Input: dimensioned drawing with shaded views. Units: mm. Origin: part minimum x, y, z. Coordinates: 2 decimals unless noted, no trailing zeros. Loops run counter-clockwise (first coordinate to the right, second up) from the corner with the lowest first, then second, coordinate; pieces in that order, holes last.
Item 1: Section A-A on z = 21. Return loops of the section in (x, y) (1 decimal).
Item 2: Ray query, line 1 along X through (y, z) = (1.5, 52); line 2 along Z through (x, y) = (35.5, 6.5) (1 decimal); line 3 along Z through (x, y) = (39, 3). Return the intervals inside material, ascending.
Item 3: Section B-B on y = 1.5. Give the number of separate pieces and of enclosed holes in the cut face.
Item 4: Section C-C on z = 96. Return loops of the section in (x, y) (1 decimal), and give its area (3 significant figures).
Item 5: Pull-direction query (Z, two-part tool) for the marked faces 1, 2 and 3; classes: released by +Z, released by -Z, zero draft, split by the parting line, or undercut.
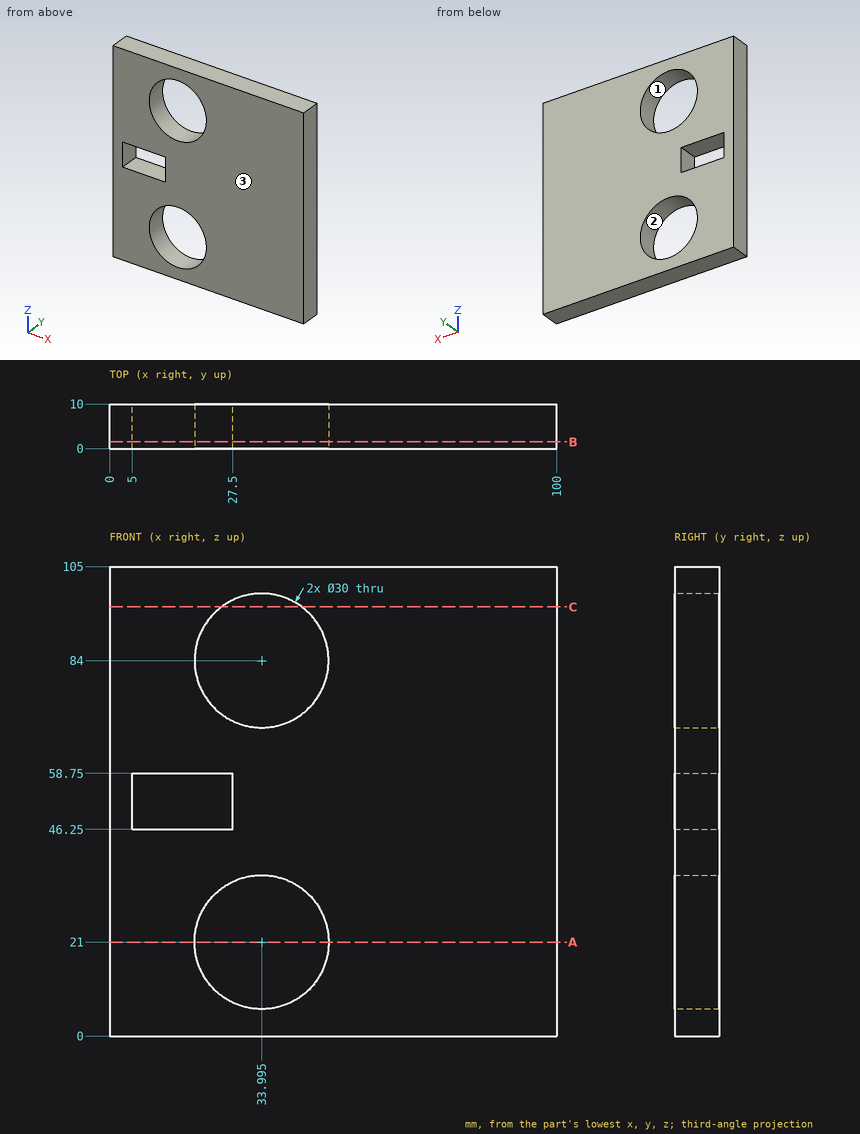
Results found:
1. outline: (0, 0) - (19, 0) - (19, 10) - (0, 10) - close; (49, 0) - (100, 0) - (100, 10) - (49, 10) - close
2. line 1: x = 0 to 5, 27.5 to 100
2. line 2: z = 0 to 6.1, 35.9 to 69.1, 98.9 to 105
2. line 3: z = 0 to 6.86, 35.14 to 69.86, 98.14 to 105
3. separate pieces: 1
3. enclosed holes: 3
4. outline: (0, 0) - (25, 0) - (25, 10) - (0, 10) - close; (43, 0) - (100, 0) - (100, 10) - (43, 10) - close
4. area: 820 mm2
5. face 1: undercut
5. face 2: undercut
5. face 3: zero draft
